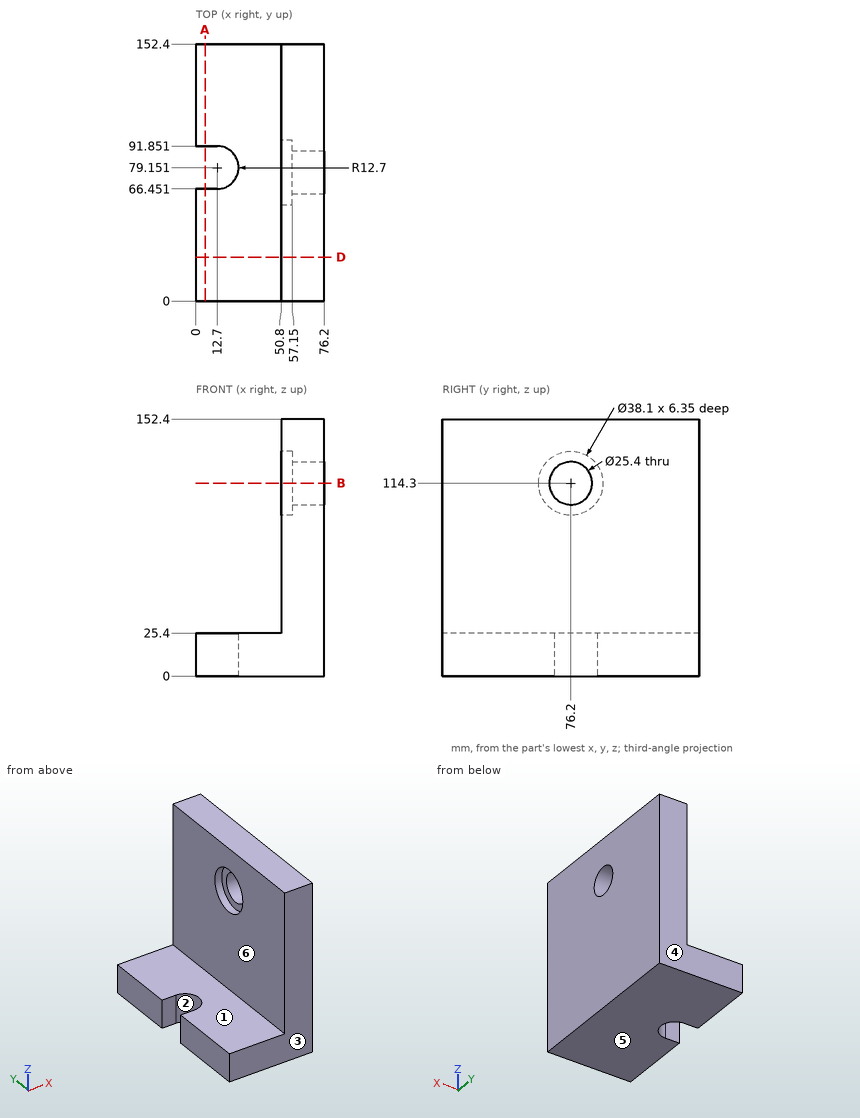
For this review, use the dimensioned drawing (mm, ordinates from the lowest corner) and the shaded views. A direction names the side the tool comes from. Coordinates: 2 decimals unless noted, no trailing zeros. Loops run counter-clockwise (first coordinate to the right, second up) from the corner with the lowest first, then second, coordinate; pieces in that order, holes last. Notation, with made-up numbers: (55, 61) - (90, 61) arc R16 cw to (90, 70) - close; hole circle Ø7 at (16, 12.25). An arc over 180 degrees is marked (long way). Use one line per item in the form item = value. Start each with the question number.
1) To check wall thickness, follow probe 1 along Z at (x, y) = (67, 76); probe 2 along Z at (x, y) = (53, 76.2); probe 3 along X at (y, z) = (10.5, 64.5). State the ranges of each line that lie inside material, in increasing order. Write a range as from..to.
2) Take a section at A-A (x = 5.5). State the section outline as (y, z) points, plus the area to 3 significant figures.
3) Take a section at B-B (z = 114.3). State the section outline as (x, y) points.
4) For the marked faces 5 and 6, list the 3-axis set-ups (+Z, -Z, +X, -X, +Y, -Y) from which the entire face can be reached by the end or side of a thin tool; tool diameter is ignored.
5) Take a section at D-D (y = 26). State the section outline as (x, z) points.
6) For pin 1 (1 mm diameter, centred on x = 43.5, y = 120, fed in from +Z), flat-tipped, find the tip position at first contact; note if it passes through.
7) Draft analysis for pull direction Y (two halves, no side actions). For the marked faces 1, 2, 3 and 4, state which applies: released by +Y, released by -Y, zero draft, split by the parting line, or undercut.
From the geometry:
q1.probe_1 = 0..101.6, 127..152.4
q1.probe_2 = 0..95.25, 133.35..152.4
q1.probe_3 = 50.8..76.2
q2.outline = (0, 0) - (66.45, 0) - (66.45, 25.4) - (0, 25.4) - close; (91.85, 0) - (152.4, 0) - (152.4, 25.4) - (91.85, 25.4) - close
q2.area = 3,230 mm2
q3.outline = (50.8, 0) - (76.2, 0) - (76.2, 63.5) - (57.15, 63.5) - (57.15, 57.15) - (50.8, 57.15) - close; (50.8, 95.25) - (57.15, 95.25) - (57.15, 88.9) - (76.2, 88.9) - (76.2, 152.4) - (50.8, 152.4) - close
q4.face_5 = -Z, +X, -X, +Y, -Y
q4.face_6 = +Z, -X, +Y, -Y
q5.outline = (0, 0) - (76.2, 0) - (76.2, 152.4) - (50.8, 152.4) - (50.8, 25.4) - (0, 25.4) - close
q6.pin_1 = 25.4
q7.face_1 = zero draft
q7.face_2 = undercut
q7.face_3 = released by -Y
q7.face_4 = released by +Y
